Input: dimensioned drawing with shaded views. Units: mm. Origin: part minimum x, y, z. A direction names the side the tool comes from. Give positions to 0.01 mm unless a question says otherwise; leave off trailing zeros. Order: outer loops, then holes, each group sorted by start corner. A loop starts at its lowest first (then second) coordinate and runs counter-clockwise, first axis right, second up. Notation, with made-up numbers: M -6,22 L 41,22 A11 ccw 41,32 Z; hole C -18,2 d5. An arc over 180 degrees is marked long. Answer in a Markdown table with one row per item. Add a question column.
(1) Section query A-A, the plane y = 238.5. Return loops of the section in (x, z) (1 decimal), plus the area to 3 significant figures.
(2) Material intervals for line 1 along Z through (x, y) = (17, 87.5) (1 decimal), sorted ascending.
(3) Pin query (flat end, axial travel): P1, Ø10.5, axis at x = 13, y = 233.5, coming from the +Z side (3 decimals); P2, Ø1, axis at x = 1, z = 35, coming from the +Y side; P3, Ø12, axis at y = 284.5, z = 14.5, coming from the +X side (3 decimals). Return the tip coordinate at first contact, or that it passes through.
(4) Section query B-B, the plane x = 23.5. Return loops of the section in (y, z) (1 decimal), plus the area to 3 significant figures.
(5) Set-up query: the marked faces 1 and 2. Return all of +Z, -Z, +X, -X, +Y, -Y with unobstructed straight access to the full face (end or side cutting, diameter ignored); none if empty.
(6) Section query C-C, the plane z = 10.5. Return loops of the section in (x, y) (1 decimal), plus the area to 3 significant figures.
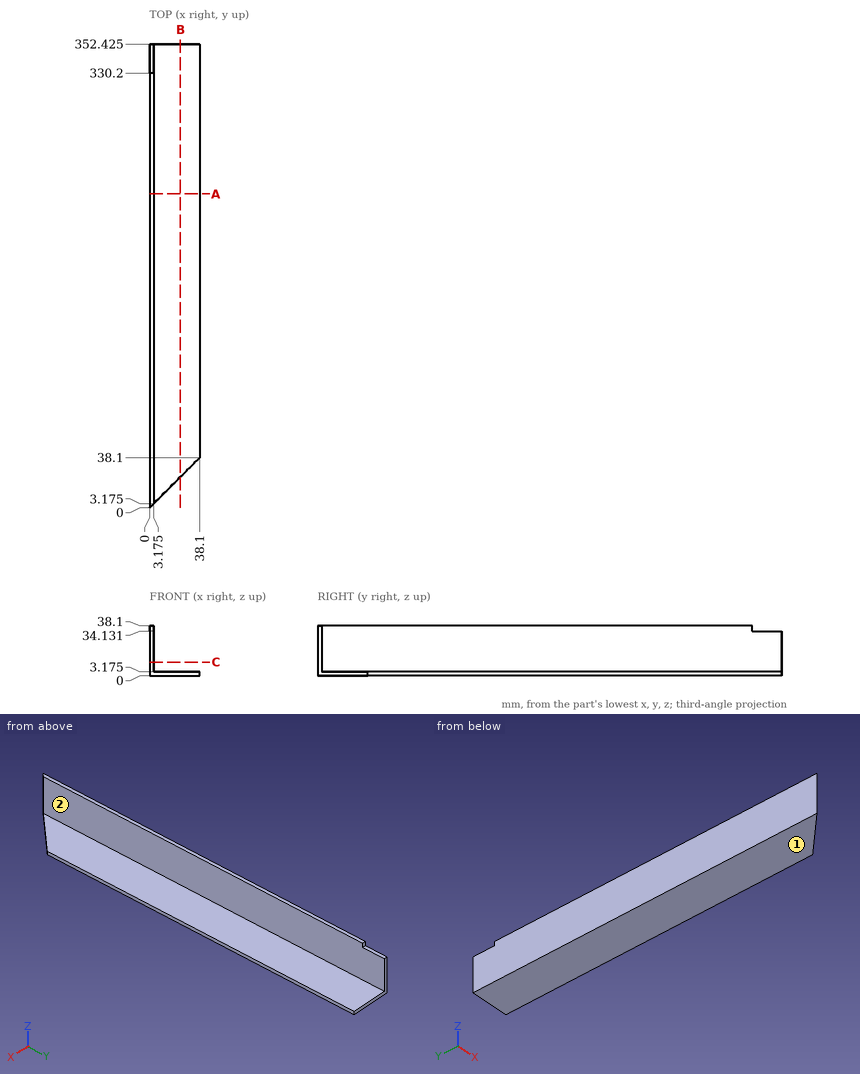
Values follow:
| question | item | result |
|---|---|---|
| 1 | outline | M 0,0 L 38.1,0 L 38.1,3.2 L 3.2,3.2 L 3.2,38.1 L 0,38.1 Z |
| 1 | area | 232 mm² |
| 2 | line 1 | z = 0 to 3.2 |
| 3 | P1 | stops at z = 3.175 |
| 3 | P2 | stops at y = 330.2 |
| 3 | P3 | stops at x = 3.175 |
| 4 | outline | M 23.5,0 L 352.4,0 L 352.4,3.2 L 23.5,3.2 Z |
| 4 | area | 1,040 mm² |
| 5 | face 1 | -Z, +X, -X, +Y, -Y |
| 5 | face 2 | +Z, +X, +Y, -Y |
| 6 | outline | M 0,0 L 3.2,3.2 L 3.2,352.4 L 0,352.4 Z |
| 6 | area | 1,110 mm² |
